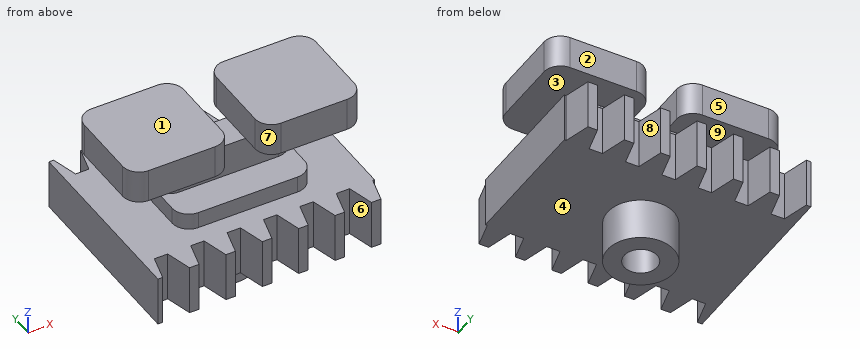
```python
from build123d import *

# Parameters (mm, degrees)
BLANKSKE_W             = 25
BLANKSKE_H             = 5.7
BLANK_DEPTH            = 3
TOOTHCUTSIM_DEPTH      = 26.816467613
TEETHCUTS_COUNT        = 12
TEETHCUTS_PITCH        = 2.199114855
MIRROR_2_COPY_1_DEPTH  = 26.816467613
MIRROR_2_COPY_2_DEPTH  = 26.816467613
MIRROR_2_COPY_3_DEPTH  = 26.816467613
MIRROR_2_COPY_4_DEPTH  = 26.816467613
MIRROR_2_COPY_5_DEPTH  = 26.816467613
MIRROR_2_COPY_6_DEPTH  = 26.816467613
MIRROR_2_COPY_7_DEPTH  = 26.816467613
MIRROR_2_COPY_8_DEPTH  = 26.816467613
MIRROR_2_COPY_9_DEPTH  = 26.816467613
MIRROR_2_COPY_10_DEPTH = 26.816467613
MIRROR_2_COPY_11_DEPTH = 26.816467613
SKETCH_2_R             = 2
EXTRUDE_1_DEPTH        = 2.5
SKETCH_3_R             = 0.5
CUT_EXTRUDE_3_DEPTH    = 27.224797425
CUT_EXTRUDE_4_DEPTH    = 10
SKETCH_6_W             = 8
SKETCH_6_H             = 2
EXTRUDE_3_DEPTH        = 3
SKETCH_7_W             = 6
SKETCH_7_H             = 6
EXTRUDE_4_DEPTH        = 2
FILLET_1_R             = 1
FILLET_2_R             = 1
SKETCH_8_W             = 8
SKETCH_8_H             = 6
EXTRUDE_5_DEPTH        = 1
FILLET_5_R             = 1
CUT_EXTRUDE_5_DEPTH    = 24.274077912
SKETCH_10_R            = 1
CUT_EXTRUDE_6_DEPTH    = 5.5


with BuildPart() as part:
    # BlankSke → Blank (new body)
    with BuildSketch(Plane.XY):
        with Locations((12.5, 2.85)):
            Rectangle(BLANKSKE_W, BLANKSKE_H)
    blank = extrude(amount=-BLANK_DEPTH)

    # TooCutSkeSim → ToothCutSim (cut, through all)
    with BuildSketch(Plane.XY):
        Polygon((0.404488327, 4.125), (-0.404488327, 4.125), (-0.818379909, 5.7254), (0.818379909, 5.7254), align=None)
    toothcutsim = extrude(amount=-TOOTHCUTSIM_DEPTH, mode=Mode.SUBTRACT)

    # TeethCuts: ToothCutSim ×12
    with Locations(*[(i * TEETHCUTS_PITCH, 0, 0) for i in range(1, TEETHCUTS_COUNT)]):
        add(toothcutsim, mode=Mode.SUBTRACT)

    # 镜向2: Blank, ToothCutSim across plane
    add(blank.mirror(Plane(origin=(0, 0, -3), x_dir=(0, 0, 1), z_dir=(0, -1, 0))))
    add(toothcutsim.mirror(Plane(origin=(0, 0, -3), x_dir=(0, 0, 1), z_dir=(0, -1, 0))), mode=Mode.SUBTRACT)

    # 镜向2 copy 1 sketch → 镜向2 copy 1 (cut, through all)
    with BuildSketch(Plane(origin=(2.199114855, 0, 0), x_dir=(1, 0, 0), z_dir=(0, 0, 1))):
        Polygon((0.404488327, -4.125), (-0.404488327, -4.125), (-0.818379909, -5.7254), (0.818379909, -5.7254), align=None)
    extrude(amount=-MIRROR_2_COPY_1_DEPTH, mode=Mode.SUBTRACT)

    # 镜向2 copy 2 sketch → 镜向2 copy 2 (cut, through all)
    with BuildSketch(Plane(origin=(4.39822971, 0, 0), x_dir=(1, 0, 0), z_dir=(0, 0, 1))):
        Polygon((0.404488327, -4.125), (-0.404488327, -4.125), (-0.818379909, -5.7254), (0.818379909, -5.7254), align=None)
    extrude(amount=-MIRROR_2_COPY_2_DEPTH, mode=Mode.SUBTRACT)

    # 镜向2 copy 3 sketch → 镜向2 copy 3 (cut, through all)
    with BuildSketch(Plane(origin=(6.597344565, 0, 0), x_dir=(1, 0, 0), z_dir=(0, 0, 1))):
        Polygon((0.404488327, -4.125), (-0.404488327, -4.125), (-0.818379909, -5.7254), (0.818379909, -5.7254), align=None)
    extrude(amount=-MIRROR_2_COPY_3_DEPTH, mode=Mode.SUBTRACT)

    # 镜向2 copy 4 sketch → 镜向2 copy 4 (cut, through all)
    with BuildSketch(Plane(origin=(8.79645942, 0, 0), x_dir=(1, 0, 0), z_dir=(0, 0, 1))):
        Polygon((0.404488327, -4.125), (-0.404488327, -4.125), (-0.818379909, -5.7254), (0.818379909, -5.7254), align=None)
    extrude(amount=-MIRROR_2_COPY_4_DEPTH, mode=Mode.SUBTRACT)

    # 镜向2 copy 5 sketch → 镜向2 copy 5 (cut, through all)
    with BuildSketch(Plane(origin=(10.995574275, 0, 0), x_dir=(1, 0, 0), z_dir=(0, 0, 1))):
        Polygon((0.404488327, -4.125), (-0.404488327, -4.125), (-0.818379909, -5.7254), (0.818379909, -5.7254), align=None)
    extrude(amount=-MIRROR_2_COPY_5_DEPTH, mode=Mode.SUBTRACT)

    # 镜向2 copy 6 sketch → 镜向2 copy 6 (cut, through all)
    with BuildSketch(Plane(origin=(13.19468913, 0, 0), x_dir=(1, 0, 0), z_dir=(0, 0, 1))):
        Polygon((0.404488327, -4.125), (-0.404488327, -4.125), (-0.818379909, -5.7254), (0.818379909, -5.7254), align=None)
    extrude(amount=-MIRROR_2_COPY_6_DEPTH, mode=Mode.SUBTRACT)

    # 镜向2 copy 7 sketch → 镜向2 copy 7 (cut, through all)
    with BuildSketch(Plane(origin=(15.393803985, 0, 0), x_dir=(1, 0, 0), z_dir=(0, 0, 1))):
        Polygon((0.404488327, -4.125), (-0.404488327, -4.125), (-0.818379909, -5.7254), (0.818379909, -5.7254), align=None)
    extrude(amount=-MIRROR_2_COPY_7_DEPTH, mode=Mode.SUBTRACT)

    # 镜向2 copy 8 sketch → 镜向2 copy 8 (cut, through all)
    with BuildSketch(Plane(origin=(17.59291884, 0, 0), x_dir=(1, 0, 0), z_dir=(0, 0, 1))):
        Polygon((0.404488327, -4.125), (-0.404488327, -4.125), (-0.818379909, -5.7254), (0.818379909, -5.7254), align=None)
    extrude(amount=-MIRROR_2_COPY_8_DEPTH, mode=Mode.SUBTRACT)

    # 镜向2 copy 9 sketch → 镜向2 copy 9 (cut, through all)
    with BuildSketch(Plane(origin=(19.792033695, 0, 0), x_dir=(1, 0, 0), z_dir=(0, 0, 1))):
        Polygon((0.404488327, -4.125), (-0.404488327, -4.125), (-0.818379909, -5.7254), (0.818379909, -5.7254), align=None)
    extrude(amount=-MIRROR_2_COPY_9_DEPTH, mode=Mode.SUBTRACT)

    # 镜向2 copy 10 sketch → 镜向2 copy 10 (cut, through all)
    with BuildSketch(Plane(origin=(21.99114855, 0, 0), x_dir=(1, 0, 0), z_dir=(0, 0, 1))):
        Polygon((0.404488327, -4.125), (-0.404488327, -4.125), (-0.818379909, -5.7254), (0.818379909, -5.7254), align=None)
    extrude(amount=-MIRROR_2_COPY_10_DEPTH, mode=Mode.SUBTRACT)

    # 镜向2 copy 11 sketch → 镜向2 copy 11 (cut, through all)
    with BuildSketch(Plane(origin=(24.190263405, 0, 0), x_dir=(1, 0, 0), z_dir=(0, 0, 1))):
        Polygon((0.404488327, -4.125), (-0.404488327, -4.125), (-0.818379909, -5.7254), (0.818379909, -5.7254), align=None)
    extrude(amount=-MIRROR_2_COPY_11_DEPTH, mode=Mode.SUBTRACT)

    # 草图2 → 凸台-拉伸1 (add)
    with BuildSketch(Plane(origin=(0, 0, -3), x_dir=(-1, 0, 0), z_dir=(0, 0, -1))):
        with Locations((-12.5, 0)):
            Circle(SKETCH_2_R)
    extrude(amount=EXTRUDE_1_DEPTH)

    # 草图3 → 切除-拉伸3 (cut, through all)
    with BuildSketch(Plane(origin=(0, 0, -5.5), x_dir=(-1, 0, 0), z_dir=(0, 0, -1))):
        with Locations((-12.5, 0)):
            Circle(SKETCH_3_R)
    extrude(amount=-CUT_EXTRUDE_3_DEPTH, mode=Mode.SUBTRACT)

    # 草图4 → 切除-拉伸4 (cut)
    with BuildSketch(Plane(origin=(0, 0, -3), x_dir=(-1, 0, 0), z_dir=(0, 0, -1))):
        Polygon((-21.884759598, 2.149584132), (-21.884759598, -2.149584132), (-21.884759598, -6.579197657), (-25.677355537, -6.579197657), (-25.677355537, 5.959830346), (-21.884759598, 5.959830346), align=None)
        Polygon((-2.5, 4.125), (-2.5, -4.125), (-2.5, -6.073591689), (0, -6.073591689), (0, 6.402235568), (-2.5, 6.402235568), align=None)
    extrude(amount=-CUT_EXTRUDE_4_DEPTH, mode=Mode.SUBTRACT)

    # 草图6 → 凸台-拉伸3 (add)
    with BuildSketch(Plane.XY):
        with Locations((12.5, 0)):
            Rectangle(SKETCH_6_W, SKETCH_6_H)
    extrude(amount=EXTRUDE_3_DEPTH)

    # 草图7 → 凸台-拉伸4 (add)
    with BuildSketch(Plane.XY.offset(3)):
        with Locations((8.5, 0)):
            Rectangle(SKETCH_7_W, SKETCH_7_H)
        with Locations((16.5, 0)):
            Rectangle(SKETCH_7_W, SKETCH_7_H)
    extrude(amount=EXTRUDE_4_DEPTH)

    # 圆角1
    fillet_1_edges = [part.edges().sort_by_distance(p)[0] for p in [
        (16.5, -1, 1.5),
        (8.5, -1, 1.5),
        (16.5, 1, 1.5),
        (8.5, 1, 1.5),
    ]]
    fillet(fillet_1_edges, radius=FILLET_1_R - 0.0001)  # a hair under: the kernel refuses the full size

    # 圆角2
    fillet_2_edges = [part.edges().sort_by_distance(p)[0] for p in [
        (5.5, 3, 4),
        (5.5, -3, 4),
        (11.5, -3, 4),
        (11.5, 3, 4),
        (19.5, 3, 4),
        (13.5, 3, 4),
        (13.5, -3, 4),
        (19.5, -3, 4),
    ]]
    fillet(fillet_2_edges, radius=FILLET_2_R)

    # 草图8 → 凸台-拉伸5 (add)
    with BuildSketch(Plane.XY):
        with Locations((12.5, 0)):
            Rectangle(SKETCH_8_W, SKETCH_8_H)
    extrude(amount=EXTRUDE_5_DEPTH)

    # 圆角5
    fillet_5_edges = [part.edges().sort_by_distance(p)[0] for p in [
        (16.5, -3, 0.5),
        (8.5, 3, 0.5),
        (16.5, 3, 0.5),
        (8.5, -3, 0.5),
    ]]
    fillet(fillet_5_edges, radius=FILLET_5_R)

    # 草图9 → 切除-拉伸5 (cut, through all)
    with BuildSketch(Plane.XY):
        Polygon((5.5, 0), (5.5, -6.223195751), (2.23821655, -6.223195751), (2.23821655, 6.249606369), (5.5, 6.249606369), align=None)
        Polygon((19.5, 0), (19.5, -6.223195751), (22.40634716, -6.223195751), (22.40634716, 6.249606369), (19.5, 6.249606369), align=None)
    extrude(amount=-CUT_EXTRUDE_5_DEPTH, mode=Mode.SUBTRACT)

    # 草图10 → 切除-拉伸6 (cut)
    with BuildSketch(Plane(origin=(0, 0, -5.5), x_dir=(-1, 0, 0), z_dir=(0, 0, -1))):
        with Locations((-12.5, 0)):
            Circle(SKETCH_10_R)
    extrude(amount=-CUT_EXTRUDE_6_DEPTH, mode=Mode.SUBTRACT)


solid = part.part
```
Input: part model. Units: mm. Frame: model coordinates. Face numbers are marked on the shaded views. A direction names the side the tool comes from. Give positions to 0.01 mm unless a question says otherwise; leave off trailing zeros. Loops run counter-clockwise (first coordinate to the right, second up) from the corner with the lowest first, then second, coordinate; pieces in that order, holes last. Notation, with made-up numbers: M 17,0.25 L 24,0.25 A24 cw 24,23.25 Z; hole C 23,-26 d1. An arc over 180 degrees is marked long. Answer as CSV lines item,"result". Start each with the question number.
1. Reachability of the marked faces 5, 6, 7, 8 and 9 from +Z, -Z, +X, -X, +Y, -Y: full face, straight path, thin tool, end or side. Return the list, or none.
2. Line query: L1, parallel to Z at x = 7.5, y = 2; L2, parallel to Y at x = 12.5, z = -3.05; L3, parallel to Z at x = 10.25, y = -4.75. Output: solid intervals per line, ascending.
3. Section D-D on z = 0.25. Return loops of the section in (x, y), plus the area to 3 significant figures.
4. Pull-direction query (Z, two-part tool) for the marked faces 1, 2, 3 and 4; classes: released by +Z, released by -Z, zero draft, split by the parting line, or undercut.
5. Section B-B on x = 17.5. Return loops of the section in (y, z) (3 decimals).
6. Pin query (flat end, axial travel): P1, Ø6.5, axis at x = 18, y = 0.5, coming from the -Z side; P2, Ø0.6, axis at x = 7.5, z = 4, coming from the +Y side. Return the tip coordinate at first contact, or that it passes through.
7. Section A-A on z = 4. Return loops of the section in (x, y).
8. Section C-C on y = -1.75. Return loops of the section in (x, z), plus the area to 3 significant figures.
Computed values:
1,face 5,"+Z, +X, -X, +Y"
1,face 6,"+Z, -Z, -Y"
1,face 7,"+Z, -Y"
1,face 8,"+Z, -Z, +Y"
1,face 9,"-X"
2,L1,"z = -3 to 0, 3 to 5"
2,L2,"y = -2 to -1, 1 to 2"
2,L3,"z = -3 to 0"
3,outline,"M 8.5,-2 A1 ccw 9.5,-3 L 15.5,-3 A1 ccw 16.5,-2 L 16.5,2 A1 ccw 15.5,3 L 9.5,3 A1 ccw 8.5,2 Z"
3,area,"47.1 mm²"
4,face 1,"released by +Z"
4,face 2,"zero draft"
4,face 3,"undercut"
4,face 4,"released by -Z"
5,outline,"M -4.125,-3 L 4.125,-3 L 4.125,0 L -4.125,0 Z; M -3,3 L 3,3 L 3,5 L -3,5 Z"
6,P1,"stops at z = -3"
6,P2,"stops at y = 3"
7,outline,"M 5.5,-2 A1 ccw 6.5,-3 L 10.5,-3 A1 ccw 11.5,-2 L 11.5,2 A1 ccw 10.5,3 L 6.5,3 A1 ccw 5.5,2 Z; M 13.5,-2 A1 ccw 14.5,-3 L 18.5,-3 A1 ccw 19.5,-2 L 19.5,2 A1 ccw 18.5,3 L 14.5,3 A1 ccw 13.5,2 Z"
8,outline,"M 5.5,-3 L 11.53,-3 L 11.53,-5.5 L 13.47,-5.5 L 13.47,-3 L 19.5,-3 L 19.5,0 L 16.5,0 L 16.5,1 L 8.5,1 L 8.5,0 L 5.5,0 Z; M 5.5,3 L 11.5,3 L 11.5,5 L 5.5,5 Z; M 13.5,3 L 19.5,3 L 19.5,5 L 13.5,5 Z"
8,area,"78.8 mm²"
